Can you work these out from the model? Positions are in its coordinate system, mm. Give positions to 0.01 mm unless a question says otherwise; leave off trailing zeros. Loops run counter-clockwise (first coordinate to the right, second up) from the corner with the lowest first, then second, coordinate; pieces in that order, holes last. Notation, with made-up numbers: (-10, 48) -> (11, 48) arc R27 ccw to (11, 70) -> close; hole circle Ø3 at (53, 8.25). An arc over 180 degrees is marked (long way). One line per question, with ' | ' between items.
Autodesk Inventor part; units mm, degrees
ref_plane "Plan YZ" through (0, 0, 0) normal (1, 0, 0) x (0, 1, 0)
ref_plane "Plan XZ" through (0, 0, 0) normal (0, 1, 0) x (-1, 0, 0)
ref_plane "Plan XY" through (0, 0, 0) normal (0, 0, 1) x (1, 0, 0)
sketch "Esquisse1" plane through (0, 0, 0) normal (0, 0, 1) x (1, 0, 0)
  line L0 (-142.5, 41.5) -> (-142.5, 37.5)
  line L1 (-142.5, 41.5) -> (-127.5, 41.5)
  line L2 (-127.5, 41.5) -> (-127.5, 37.5)
  line L3 (0, -58.1) -> (0, 58.1) construction
  line L4 (-206.5, 0) -> (206.5, 0) construction
  line L5 (-75, 41.5) -> (-75, 37.5)
  line L6 (-75, 41.5) -> (-60, 41.5)
  line L7 (-60, 41.5) -> (-60, 37.5)
  line L8 (-7.5, 41.5) -> (-7.5, 37.5)
  line L9 (-7.5, 41.5) -> (7.5, 41.5)
  line L10 (7.5, 41.5) -> (7.5, 37.5)
  line L11 (60, 41.5) -> (60, 37.5)
  line L12 (60, 41.5) -> (75, 41.5)
  line L13 (75, 41.5) -> (75, 37.5)
  line L14 (127.5, 41.5) -> (127.5, 37.5)
  line L15 (127.5, 41.5) -> (142.5, 41.5)
  line L16 (142.5, 41.5) -> (142.5, 37.5)
  line L17 (-127.5, 37.5) -> (-75, 37.5)
  line L18 (-60, 37.5) -> (-7.5, 37.5)
  line L19 (7.5, 37.5) -> (60, 37.5)
  line L20 (75, 37.5) -> (127.5, 37.5)
  line L21 (142.5, 37.5) -> (147.5, 37.5)
  line L22 (-142.5, 37.5) -> (-147.5, 37.5)
  line L23 (-142.5, -41.5) -> (-142.5, -37.5)
  line L24 (-142.5, -41.5) -> (-127.5, -41.5)
  line L25 (-127.5, -41.5) -> (-127.5, -37.5)
  line L26 (-75, -41.5) -> (-75, -37.5)
  line L27 (-75, -41.5) -> (-60, -41.5)
  line L28 (-60, -41.5) -> (-60, -37.5)
  line L29 (-7.5, -41.5) -> (-7.5, -37.5)
  line L30 (-7.5, -41.5) -> (7.5, -41.5)
  line L31 (7.5, -41.5) -> (7.5, -37.5)
  line L32 (60, -41.5) -> (60, -37.5)
  line L33 (60, -41.5) -> (75, -41.5)
  line L34 (75, -41.5) -> (75, -37.5)
  line L35 (127.5, -41.5) -> (127.5, -37.5)
  line L36 (127.5, -41.5) -> (142.5, -41.5)
  line L37 (142.5, -41.5) -> (142.5, -37.5)
  line L38 (-127.5, -37.5) -> (-75, -37.5)
  line L39 (-60, -37.5) -> (-7.5, -37.5)
  line L40 (7.5, -37.5) -> (60, -37.5)
  line L41 (75, -37.5) -> (127.5, -37.5)
  line L42 (142.5, -37.5) -> (147.5, -37.5)
  line L43 (-142.5, -37.5) -> (-147.5, -37.5)
  line L44 (147.5, -37.5) -> (147.5, 37.5)
  line L45 (-147.5, -37.5) -> (-147.5, 37.5)
  point P0 (0, 0)
  dimension "d1" = 15
  dimension "d2" = 4
  dimension "d3" = 4
  dimension "d6" = 67.5
  dimension "d11" = 5
  dimension "d12" = 5
  dimension "d30" = 75
extrude "Extrusion1" add sketch "Esquisse1" along normal blind 4
sketch "Esquisse6" plane through (0, 0, 4) normal (0, 0, 1) x (1, 0, 0)
  line L0 (0, -58.1) -> (0, 58.1) construction
  line L1 (-206.5, 0) -> (206.5, 0) construction
  point P0 (0, 0)
  point P1 (-142.5, 37.5)
  point P2 (-127.5, 37.5)
  point P3 (-75, 37.5)
  point P4 (-60, 37.5)
  point P5 (-7.5, 37.5)
  point P6 (7.5, 37.5)
  point P7 (60, 37.5)
  point P8 (75, 37.5)
  point P9 (142.5, 37.5)
  point P10 (127.5, 37.5)
  point P11 (-142.5, -37.5)
  point P12 (-127.5, -37.5)
  point P13 (-75, -37.5)
  point P14 (-60, -37.5)
  point P15 (-7.5, -37.5)
  point P16 (7.5, -37.5)
  point P17 (60, -37.5)
  point P18 (75, -37.5)
  point P19 (142.5, -37.5)
  point P20 (127.5, -37.5)
hole "Perçage1" at (-142.5, 37.5, 4) at (-127.5, 37.5, 4) at (-75, 37.5, 4) at (-60, 37.5, 4) at (-7.5, 37.5, 4) at (7.5, 37.5, 4) at (60, 37.5, 4) at (75, 37.5, 4) at (142.5, 37.5, 4) at (127.5, 37.5, 4) at (127.5, -37.5, 4) at (142.5, -37.5, 4) at (75, -37.5, 4) at (60, -37.5, 4) at (7.5, -37.5, 4) at (-7.5, -37.5, 4) at (-60, -37.5, 4) at (-75, -37.5, 4) at (-127.5, -37.5, 4) at (-142.5, -37.5, 4) direction (0, 0, -1) diameter 1 end through all
chamfer "Chanfrein1" distance 1 angle 45 20 edges at (-142.5, 41.5, 2) (-127.5, 41.5, 2) (-75, 41.5, 2) (-60, 41.5, 2) (-7.5, 41.5, 2) (7.5, 41.5, 2) (60, 41.5, 2) (75, 41.5, 2) (127.5, 41.5, 2) (142.5, 41.5, 2) (142.5, -41.5, 2) (127.5, -41.5, 2) (60, -41.5, 2) (75, -41.5, 2) (-142.5, -41.5, 2) (-127.5, -41.5, 2) (-75, -41.5, 2) (-60, -41.5, 2) (-7.5, -41.5, 2) (7.5, -41.5, 2)
sketch "Esquisse10" plane through (0, 0, 4) normal (0, 0, 1) x (1, 0, 0)
  line L0 (0, -58.1) -> (0, 58.1) construction
  line L1 (-206.5, 0) -> (206.5, 0) construction
  line L2 (-115, 5.5) -> (-95, 5.5)
  line L3 (-95, 5.5) -> (-95, -5.5)
  line L4 (-95, -5.5) -> (-115, -5.5)
  line L5 (-115, -5.5) -> (-115, 5.5)
  dimension "d61" = 95
  dimension "d62" = 20
  dimension "d63" = 11
sketch "Esquisse11" plane through (0, 0, 4) normal (0, 0, 1) x (1, 0, 0)
  line L0 (-206.5, 0) -> (206.5, 0) construction
  point P0 (0, 0)
  point P1 (-117.494, 0)
  point P2 (-92.5, 0)
  dimension "d66" = 24.994
  dimension "d69" = 92.5
extrude "Extrusion4" cut sketch "Esquisse10" against normal blind 10
hole "Perçage5" at (-117.494, 0, 4) at (-92.5, 0, 4) direction (0, 0, -1) diameter 2.459 end through all
properties part number "P1704_004" material "Plastique PMMA"
Q1. For pin 1 Ø0.8 at (y, z) = (-39.5, 2) entering from -X; pin 2 Ø2 at (x, z) = (-105, 1.5) entering from -Y; pin 3 Ø0.8 at (y, z) = (39.5, 2) entering from +X, each with a flat end and sliding along its axis, tell me the tip position at first contact or that it passes through.
Entries:
pin 1: x = -142.5 | pin 2: y = -37.5 | pin 3: x = 142.5
Q2. If I drill on probe 1 along X at (y, z) = (0, 1.55); probe 2 along Y at (x, z) = (-104.5, 1.2); probe 3 along X at (y, z) = (1.5, 0.65), over which ranges is the centre line in solid material (lowest first)? Write a range as from..to.
Entries:
probe 1: -147.5..-118.72, -116.26..-115, -95..-93.73, -91.27..147.5 | probe 2: -37.5..-5.5, 5.5..37.5 | probe 3: -147.5..-115, -95..147.5
Q3. If we section it at A-A (x = -18): Write out the boundary of the cut face in (y, z).
Entries:
outline: (-37.5, 0) -> (37.5, 0) -> (37.5, 4) -> (-37.5, 4) -> close
Q4. If we section it at B-B (z = 3.1): State how many separate pieces and enclosed holes the cut face has, plus the area to 3 significant figures.
Entries:
separate pieces: 1 | enclosed holes: 3 | area: 22,500 mm²
